from build123d import *

# Parameters (mm, degrees)
SKETCH_W        = 102
SKETCH_H        = 44.5
PAD_DEPTH       = 16
SKETCH001_W     = 97.5
SKETCH001_H     = 40.5
POCKET_DEPTH    = 14
SKETCH002_R     = 3
PAD001_DEPTH    = 15
SKETCH007_R     = 1.25
POCKET004_DEPTH = 35
SKETCH008_R     = 2.375
POCKET005_DEPTH = 27
POCKET008_DEPTH = 5
SKETCH012_R     = 4.5
POCKET009_DEPTH = 10
SKETCH013_R     = 7
POCKET010_DEPTH = 1.2
SKETCH022_W     = 2.5
SKETCH022_H     = 44.5
POCKET018_DEPTH = 13
POCKET019_DEPTH = 2
POCKET020_DEPTH = 14


with BuildPart() as part:
    # Sketch → Pad (new body)
    with BuildSketch(Plane.XY):
        with Locations((51, 22.25)):
            Rectangle(SKETCH_W, SKETCH_H)
    extrude(amount=PAD_DEPTH)

    # Sketch001 (on Face6 of Pad) → Pocket (cut)
    with BuildSketch(Plane.XY.offset(16)):
        with Locations((51.25, 22.25)):
            Rectangle(SKETCH001_W, SKETCH001_H)
    extrude(amount=-POCKET_DEPTH, mode=Mode.SUBTRACT)

    # Sketch002 (on Face11 of Pocket) → Pad001 (join)
    with BuildSketch(Plane.XY.offset(2)):
        with Locations((6.5, 39.75)):
            Circle(SKETCH002_R)
        with Locations((97, 39.75)):
            Circle(SKETCH002_R)
        with Locations((6.5, 4.75)):
            Circle(SKETCH002_R)
        with Locations((97, 4.75)):
            Circle(SKETCH002_R)
    extrude(amount=PAD001_DEPTH)

    # Sketch007 (on DatumPlane) → Pocket004 (cut)
    with BuildSketch(Plane(origin=(0, 0, -18), x_dir=(1, 0, 0), z_dir=(0, 0, -1))):
        with Locations((6.5, -4.75)):
            Circle(SKETCH007_R)
        with Locations((97, -4.75)):
            Circle(SKETCH007_R)
        with Locations((6.5, -39.75)):
            Circle(SKETCH007_R)
        with Locations((97, -39.75)):
            Circle(SKETCH007_R)
    extrude(amount=-POCKET004_DEPTH, mode=Mode.SUBTRACT)

    # Sketch008 (on DatumPlane) → Pocket005 (cut)
    with BuildSketch(Plane(origin=(0, 0, -18), x_dir=(1, 0, 0), z_dir=(0, 0, -1))):
        with Locations((6.5, -4.75)):
            Circle(SKETCH008_R)
        with Locations((97, -4.75)):
            Circle(SKETCH008_R)
        with Locations((6.5, -39.75)):
            Circle(SKETCH008_R)
        with Locations((97, -39.75)):
            Circle(SKETCH008_R)
    extrude(amount=-POCKET005_DEPTH, mode=Mode.SUBTRACT)

    # Sketch011 → Pocket008 (cut)
    with BuildSketch(Plane.YZ.offset(102)):
        with BuildLine():
            ThreePointArc((18.5, 7), (16.5, 5), (18.5, 3))
            Line((18.5, 3), (25.5, 3))
            ThreePointArc((25.5, 3), (27.5, 5), (25.5, 7))
            Line((25.5, 7), (18.5, 7))
        make_face()
    extrude(amount=-POCKET008_DEPTH, mode=Mode.SUBTRACT)

    # Sketch012 (on Face1 of Pocket008) → Pocket009 (cut)
    with BuildSketch(Plane.XZ):
        with Locations((45, 14)):
            Circle(SKETCH012_R)
    extrude(amount=-POCKET009_DEPTH, mode=Mode.SUBTRACT)

    # Sketch013 (on Face17 of Pocket009) → Pocket010 (cut)
    with BuildSketch(Plane(origin=(0, 2, 0), x_dir=(-1, 0, 0), z_dir=(0, 1, 0))):
        with Locations((-45, 14)):
            Circle(SKETCH013_R)
    extrude(amount=-POCKET010_DEPTH, mode=Mode.SUBTRACT)

    # Sketch022 → Pocket018 (cut)
    with BuildSketch(Plane.XY.offset(16)):
        with Locations((1.25, 22.25)):
            Rectangle(SKETCH022_W, SKETCH022_H)
    extrude(amount=-POCKET018_DEPTH, mode=Mode.SUBTRACT)

    # Sketch023 (on Face4 of Pocket018) → Pocket019 (cut)
    with BuildSketch(Plane.XY.offset(16)):
        Polygon((2.499048, 44.5), (102, 44.5), (102, 0), (2.5, 0), (2.5, 0.8), (101.2, 0.8), (101.2, 43.7), (2.499048, 43.7), align=None)
    extrude(amount=-POCKET019_DEPTH, mode=Mode.SUBTRACT)

    # Sketch024 (on Face25 of Pocket019) → Pocket020 (cut)
    with BuildSketch(Plane.XY.offset(16)):
        Polygon((4.163707, 0), (4.163707, 0.8), (0.800622, 0.8), (0.800622, 43.7), (4.5, 43.7), (4.5, 44.5), (0, 44.5), (0, 0), align=None)
    extrude(amount=-POCKET020_DEPTH, mode=Mode.SUBTRACT)


solid = part.part
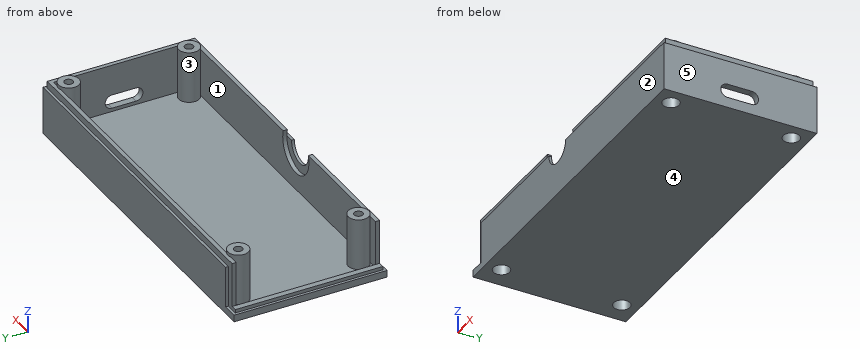
The listing builds one solid part. Answer for the finished solid, in the listing's coordinates (mm). Face numbers are marked on the shaded views. A direction names the side the tool comes from. Coordinates: 2 decimals unless noted, no trailing zeros. Order: outer loops, then holes, each group sorted by start corner. A loop starts at its lowest first (then second) coordinate and runs counter-clockwise, first axis right, second up.
Q1. A cutting plane is placed at C-C, the plane x = 16.5. Write down the section's boundary in (y, z).
Q2. Which of the six approach directions +Z, -Z, +X, -X, +Y, -Y give full straight-line access (tool end or side, diameter ignored) to the marked faces 1 and 2?
Q3. For a pull along X with two mould halves and no side action, classify the marked faces 3, 4 and 5 as pulls with the +X half, pulls with the -X half, needs draft (parallel to the pull), parting line crosses it, or undercut.
Q4. Consider line 1 (Y direction, x = 97, z = 6) (3 decimals); line 2 (X direction, y = 37, z = 7); line 3 (Y direction, x = 20, z = 6). Determine where each line is inside the solid, lowest interval first.
Q5. Given P1, Ø4, axis at x = 6.5, y = 39.75, coming from the -Z side; P2, Ø1.5, axis at x = 44, y = 38, coming from the +Z side; P3, Ø1, axis at x = 101, y = 22, coming from the +Z side, each flat-ended and moving along its own axis, determine where each tip first touches the part or whether it passes through.
Answers follow:
1. outline: (0, 0) - (44.5, 0) - (44.5, 14) - (43.7, 14) - (43.7, 16) - (42.5, 16) - (42.5, 2) - (2, 2) - (2, 16) - (0.8, 16) - (0.8, 14) - (0, 14) - close
2. face 1: +Z
2. face 2: +Z, -Z, +X, -X, -Y
3. face 3: undercut
3. face 4: needs draft
3. face 5: pulls with the +X half
4. line 1: y = 0 to 2.375, 7.125 to 7.75, 36.75 to 37.375, 42.125 to 44.5
4. line 2: x = 5.3 to 7.7, 95.8 to 98.2, 100 to 102
4. line 3: y = 0 to 2, 42.5 to 44.5
5. P1: stops at z = 9
5. P2: stops at z = 2
5. P3: stops at z = 16
